Could you check a few things on this model? Use its own coordinates, in mm. A direction names the side the tool comes from. Round coordinates to 2 decimals unless told otherwise and drop trailing zeros. Loops run counter-clockwise (first coordinate to the right, second up) from the corner with the lowest first, then second, coordinate; pieces in that order, holes last. Notation, with made-up numbers: (50.25, 16) - (67.25, 16) arc R26 cw to (67.25, 45) - close; hole circle Ø6 at (4, 26). An arc over 180 degrees is marked (long way). Use one line per item in the form item = value.
```python
from build123d import *

# Parameters (mm, degrees)
SKETCH1_R           = 12.5
BOSS_EXTRUDE1_DEPTH = 59
SKETCH2_R           = 1.575
CUT_EXTRUDE1_DEPTH  = 12.7
SKETCH3_R           = 3
BOSS_EXTRUDE2_DEPTH = 15


with BuildPart() as part:
    # Sketch1 → Boss-Extrude1 (new body)
    with BuildSketch(Plane.XY):
        with Locations((-10.391437804, 5.875911401)):
            Circle(SKETCH1_R)
    extrude(amount=BOSS_EXTRUDE1_DEPTH)

    # Sketch2 → Cut-Extrude1 (cut)
    with BuildSketch(Plane.XY.offset(59)):
        with Locations((-10.391437804, 14.397611401)):
            Circle(SKETCH2_R)
        with Locations(Location((-10.391437804, -2.645788599, 0), (0, 0, 180))):
            Circle(SKETCH2_R)
    extrude(amount=-CUT_EXTRUDE1_DEPTH, mode=Mode.SUBTRACT)

    # Sketch3 → Boss-Extrude2 (add)
    with BuildSketch(Plane.XY.offset(59)):
        with Locations((-10.391437804, 5.875911401)):
            Circle(SKETCH3_R)
    extrude(amount=BOSS_EXTRUDE2_DEPTH)


solid = part.part
```
1. We'd pull the mould along X, two halves only. Please class faces 3 (the face through (-11, 6, 0)), 4 (the face through (-10, -3, 46.3)), 5 (the face through (-7.62, 4.73, 66.4)), 6 (the face through (-10, 14, 46.3)): +X half, -X half, draft (parallel to the pull), parting line (faces both ways), or undercut.
Solution:
face_3 = draft
face_4 = undercut
face_5 = parting line
face_6 = undercut
2. For P1, Ø12, axis at y = 13, z = 42, coming from the -X side; P2, Ø3, axis at x = -10.39, y = -2.65, coming from the +Z side; P3, Ø3, axis at y = -2, z = 43.5, coming from the -X side, each with a flat end and sliding along its axis, tell me the tip position at first contact or that it passes through.
Solution:
P1 = -22.84
P2 = 46.3
P3 = -21.14
3. Please list where these lines run through material, in increasing order: line 1 along Z through (x, y) = (-4.25, 9); line 2 along Y through (x, z) = (-9, 47.5); line 3 along X through (y, z) = (13.5, 55).
Solution:
line_1 = 0 to 59
line_2 = -6.55 to -3.38, -1.91 to 13.66, 15.14 to 18.3
line_3 = -20.3 to -11.69, -9.1 to -0.49
4. If we section it at D-D, the plane x = -1: Write out the boundary of the cut face in (y, z).
Solution:
outline = (-2.37, 0) - (14.13, 0) - (14.13, 59) - (-2.37, 59) - close
5. If we section it at B-B, the plane x = -11.25: Write out the boundary of the cut face in (y, z).
Solution:
outline = (-6.59, 0) - (18.35, 0) - (18.35, 59) - (15.72, 59) - (15.72, 46.3) - (13.08, 46.3) - (13.08, 59) - (8.75, 59) - (8.75, 74) - (3, 74) - (3, 59) - (-1.33, 59) - (-1.33, 46.3) - (-3.97, 46.3) - (-3.97, 59) - (-6.59, 59) - close
6. If we section it at C-C, the plane z = 25: Write out the boundary of the cut face in (x, y).
Solution:
outline = circle Ø25 at (-10.39, 5.88)
7. On a 3-axis mill with a long thin cutter (end or side, diameter ignored), from which of +Z, -Z, +X, -X, +Y, -Y can I reach the whole of each face in a straight line? I mean faces 1 (the face through (-10, 6, 74)), 2 (the face through (-8.9, 14.9, 52.7)). Say none if no direction works.
Solution:
face_1 = +Z, +X, -X, +Y, -Y
face_2 = +Z
8. If we section it at A-A, the plane y = 8: Write out the boundary of the cut face in (x, z), plus the area to 3 significant figures.
Solution:
outline = (-22.71, 0) - (1.93, 0) - (1.93, 59) - (-8.27, 59) - (-8.27, 74) - (-12.51, 74) - (-12.51, 59) - (-22.71, 59) - close
area = 1,520 mm^2
